```python
from build123d import *

# Parameters (mm, degrees)
F1_DEPTH    = 101.6
F2_T1_DEPTH = 288.460768654
F4_START    = 84.582
F3_W        = 46.8034986407
F3_H        = 78.1666617841
F4_DEPTH    = 39.37
F6_DEPTH    = 76.2


# Not quite as in the source:
# - a fillet or chamfer that OpenCascade refuses, or shapes differently, is made with other operations: its cross-section is extruded or revolved along the edge and cut away or added


with BuildPart() as f1:
    # F0 (on Front) → F1 (new body)
    with BuildSketch(Plane.XZ):
        Polygon((-46.8246676028, -52.1724224091), (51.9963987172, -52.1724224091), (51.9963987172, 123.2375688851), (19.8580101132, 123.2375688851), (19.8580101132, -24.3260078132), (-46.8246676028, -24.3260078132), align=None)
    extrude(amount=F1_DEPTH)

    # F2: fillet of radius 52.1228708116 on 2 edges, made by hand

    # F2_s2 → F2_t1 (cut)
    with BuildSketch(Plane.XY.offset(-182.4795994381)):
        with BuildLine():
            ThreePointArc((-46.8246676028, -52.1228708116), (-31.558232197, -15.2664354058), (5.2982032089, 0))
            Line((5.2982032089, 0), (-46.8246676028, 0))
            Line((-46.8246676028, 0), (-46.8246676028, -52.1228708116))
        make_face()
        with BuildLine():
            ThreePointArc((-46.8246676028, -49.4771291884), (-31.558232197, -86.3335645942), (5.2982032089, -101.6))
            Line((5.2982032089, -101.6), (-46.8246676028, -101.6))
            Line((-46.8246676028, -101.6), (-46.8246676028, -49.4771291884))
        make_face()
    extrude(amount=F2_T1_DEPTH, mode=Mode.SUBTRACT)

    # F3 (on Front) → F4 (cut)
    with BuildSketch(Plane.XZ.offset(F4_START)):
        with Locations((39.5658416674, -25.9385192767)):
            Rectangle(F3_W, F3_H)
    extrude(amount=F4_DEPTH, mode=Mode.SUBTRACT)

    # F5 (on Right) → F6 (cut, symmetric)
    with BuildSketch(Plane.YZ):
        with BuildLine():
            Line((-29.9497395754, 125.8109509945), (-64.9317279458, 125.8109509945))
            Line((-64.9317279458, 125.8109509945), (-64.9317279458, 46.6792732477))
            ThreePointArc((-64.9317279458, 46.6792732477), (-47.4407337606, 61.9233160809), (-29.9497395754, 46.6792732477))
            Line((-29.9497395754, 46.6792732477), (-29.9497395754, 125.8109509945))
        make_face()
        with BuildLine():
            ThreePointArc((-29.9497395754, 46.6792732477), (-47.4407337606, 61.9233160809), (-64.9317279458, 46.6792732477))
            ThreePointArc((-64.9317279458, 46.6792732477), (-48.6498471956, 26.6515784611), (-29.7841407761, 44.2667230964))
            ThreePointArc((-29.7841407761, 44.2667230964), (-29.8255891253, 45.4758365314), (-29.9497395754, 46.6792732477))
        make_face()
    extrude(amount=F6_DEPTH, both=True, mode=Mode.SUBTRACT)


solid = f1.part
```
Check sheet for the modelled part. Datum: model origin and axes. Units: mm. A direction names the side the tool comes from. Round coordinates to 2 decimals unless told otherwise and drop trailing zeros. Order: outer loops, then holes, each group sorted by start corner. A loop starts at its lowest first (then second) coordinate and runs counter-clockwise, first axis right, second up. Notation, with made-up numbers: (-37.5, -3.75) -> (-1.5, -3.75) arc R10 ccw to (-1.5, 5.25) -> close; hole circle Ø5 at (56.25, 11). An arc over 180 degrees is marked (long way). One line per item, written item: value. Start each with the question number.
Q1. Cross-section at D-D (y = -94). Record the boundary of the cut face in (x, z), and give its area (3 significant figures).
Q2. Thickness scan on line 1 (Y direction, x = 30, z = 46.5); line 2 (Y direction, x = 27, z = 90.5); line 3 (Y direction, x = 31, z = 1). Record the ranges inside material, lowest first.
Q3. Cross-section at A-A (z = 112). Record the boundary of the cut face in (x, y), and give its area (3 significant figures).
Q4. Mould release check, pull along Y, two halves, no side actions. Record for faces 6 (the face through (-31.49, -15.2, -38.44)), 7 (the face through (36, -64.932, 85)), 8 (the face through (51.996, -50, 15)): pulls with the +Y half, pulls with the -Y half, needs draft (parallel to the pull), parting line crosses it, or undercut.
Q5. Set-up check for faces 1 (the face through (34, -84.582, -19)), 2 (the face through (36, -29.95, 84)), 3 (the face through (19.858, -28, 50)), 4 (the face through (36, -93, 13.145)), 5 (the face through (16.164, -93, -38)): record each of +Z, -Z, +X, -X, +Y, -Y from which the full face is reachable in a straight line by a thin tool's end or side.
Q6. Gauge pin test, flat ends, axial feed: pin 1 Ø8.5 at (x, y) = (34.5, -89) entering from -Z; pin 2 Ø1.5 at (x, y) = (-4, -85) entering from +Z; pin 3 Ø18 at (x, z) = (39, -8) entering from -Y. Record the tip position at first contact, or that the pin passes through.
Q7. Cross-section at B-B (z = -34). Record the boundary of the cut face in (x, y), and give its area (3 significant figures).
Q8. Cross-section at C-C (x = 27.5). Record the boundary of the cut face in (y, z).
Completed:
1. outline: (-21.8, -52.17) -> (16.16, -52.17) -> (16.16, -24.33) -> (-21.8, -24.33) -> close; (19.86, 13.14) -> (52, 13.14) -> (52, 123.24) -> (19.86, 123.24) -> close
1. area: 4,600 mm²
2. line 1: y = -101.6 to -64.96, -29.93 to 0
2. line 2: y = -101.6 to -64.93, -29.95 to 0
2. line 3: y = -84.58 to 0
3. outline: (19.86, -101.6) -> (52, -101.6) -> (52, -64.93) -> (19.86, -64.93) -> close; (19.86, -29.95) -> (52, -29.95) -> (52, 0) -> (19.86, 0) -> close
3. area: 2,140 mm²
4. face 6: pulls with the +Y half
4. face 7: undercut
4. face 8: needs draft
5. face 1: -Z, +X, -Y
5. face 2: +Z, +X, -X
5. face 3: +Z, -X, +Y, -Y
5. face 4: -Z, +X, -X, -Y
5. face 5: +Z, -Z, +X, -Y
6. pin 1: stops at z = 13.14
6. pin 2: stops at z = -24.33
6. pin 3: stops at y = -84.58
7. outline: (-46.81, -50.8) arc R52.12 ccw to (5.3, -101.6) -> (16.16, -101.6) -> (16.16, -84.58) -> (52, -84.58) -> (52, 0) -> (5.3, 0) arc R52.12 ccw to start
7. area: 8,260 mm²
8. outline: (-101.6, 13.14) -> (-84.58, 13.14) -> (-84.58, -52.17) -> (0, -52.17) -> (0, 123.24) -> (-29.95, 123.24) -> (-29.95, 46.68) arc R17.66 cw (long way) to (-64.93, 46.68) -> (-64.93, 123.24) -> (-101.6, 123.24) -> close
